Here's how the part is built. I have some questions about the finished solid (model axes, mm). Face numbers are marked on the shaded views. Round coordinates to 2 decimals unless told otherwise and drop trailing zeros. Loops run counter-clockwise (first coordinate to the right, second up) from the corner with the lowest first, then second, coordinate; pieces in that order, holes last. Notation, with made-up numbers: M -12,-16.75 L 20,-16.75 A19 ccw 20,-9.75 Z; hole C 6.5,84 d8. An arc over 180 degrees is marked long. Use a Markdown table: item, result.
```python
from build123d import *

# Parameters (mm, degrees)
SKETCH1_W           = 43.6
SKETCH1_H           = 20
BOSS_EXTRUDE1_DEPTH = 3
SKETCH4_R           = 14
CUT_EXTRUDE1_DEPTH  = 4
FILLET1_R           = 5
SKETCH3_W           = 3
SKETCH3_H           = 5
BOSS_EXTRUDE2_DEPTH = 3
LPATTERN1_COUNT     = 2
LPATTERN1_PITCH     = 30


with BuildPart() as part:
    # Sketch1 → Boss-Extrude1 (new body)
    with BuildSketch(Plane(origin=(0, 0, 0), x_dir=(0, 0, -1), z_dir=(1, 0, 0))):
        with Locations((-8.2, -1.75)):
            Rectangle(SKETCH1_W, SKETCH1_H)
    extrude(amount=BOSS_EXTRUDE1_DEPTH)

    # Sketch4 → Cut-Extrude1 (cut, through all)
    with BuildSketch(Plane(origin=(3, 0, 0), x_dir=(0, 0, -1), z_dir=(1, 0, 0))):
        with Locations((-8.2, 8.25)):
            Circle(SKETCH4_R)
    extrude(amount=-CUT_EXTRUDE1_DEPTH, mode=Mode.SUBTRACT)

    # Fillet1
    fillet1_edges = [part.edges().sort_by_distance(p)[0] for p in [
        (1.5, 8.25, 30),
        (1.5, 8.25, -13.6),
    ]]
    fillet(fillet1_edges, radius=FILLET1_R)

    # Sketch3 → Boss-Extrude2 (add)
    with BuildSketch(Plane.XZ.offset(11.75)):
        with Locations((1.5, 25)):
            Rectangle(SKETCH3_W, SKETCH3_H)
    boss_extrude2 = extrude(amount=BOSS_EXTRUDE2_DEPTH)

    # LPattern1: Boss-Extrude2 ×2
    with Locations(*[(0, 0, -i * LPATTERN1_PITCH) for i in range(1, LPATTERN1_COUNT)]):
        add(boss_extrude2)


solid = part.part
```
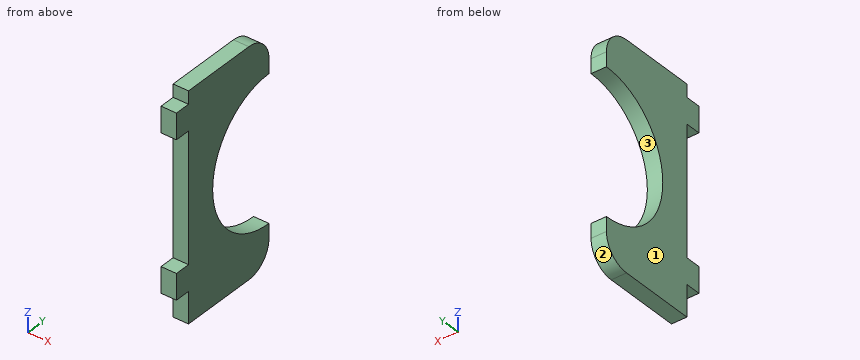
Q1. Imagine slicing it at C-C, the plane z = 8.2. Please give me the cut outline in (x, y), then the cut area to 3 significant figures.
Return value:
| item | result |
|---|---|
| outline | M 0,-11.75 L 3,-11.75 L 3,-5.75 L 0,-5.75 Z |
| area | 18.0 mm^2 |
Q2. We'd pull the mould along Z, two halves only. Please class the marked faces 1, 2 and 3: pulls with the +Z half, pulls with the -Z half, needs draft (parallel to the pull), parting line crosses it, or undercut.
Return value:
| item | result |
|---|---|
| face 1 | needs draft |
| face 2 | pulls with the -Z half |
| face 3 | undercut |
Q3. Imagine slicing it at D-D, the plane z = 16. Please give me the cut outline in (x, y).
Return value:
| item | result |
|---|---|
| outline | M 0,-11.75 L 3,-11.75 L 3,-3.38 L 0,-3.38 Z |
Q4. Will these pins go through, and if not, where does the flat tip stop? P1, Ø0.9, axis at x = 1.5, y = -13.5, coming from the +Z side; P2, Ø6, axis at y = 0.5, z = 18.5, coming from the +X side; P3, Ø1.5, axis at x = 2, z = 4, coming from the -Y side.
Return value:
| item | result |
|---|---|
| P1 | stops at z = 27.5 |
| P2 | stops at x = 3 |
| P3 | stops at y = -11.75 |
Q5. I need wall thicknesses on line 1 (Z direction, x = 0.3, y = 2.75); line 2 (Z direction, x = 1.5, y = -0.5); line 3 (Y direction, x = 0.8, z = -12). Which ranges of each line are inside material? Lowest first, please. Write a range as from..to.
Return value:
| item | result |
|---|---|
| line 1 | z = -13.6..-4.67, 21.07..30 |
| line 2 | z = -13.6..-2.73, 19.13..30 |
| line 3 | y = -11.75..6.92 |
Q6. Imagine slicing it at B-B, the plane y = -2.5. Please give me the cut outline in (x, z).
Return value:
| item | result |
|---|---|
| outline | M 0,-13.6 L 3,-13.6 L 3,-0.77 L 0,-0.77 Z; M 0,17.17 L 3,17.17 L 3,30 L 0,30 Z |
Q7. Imagine slicing it at A-A, the plane x = 0.4. Please give me the cut outline in (y, z), then the cut area to 3 significant figures.
Return value:
| item | result |
|---|---|
| outline | M -14.75,-7.5 L -11.75,-7.5 L -11.75,-13.6 L 3.25,-13.6 A5 ccw 8.25,-8.6 L 8.25,-5.8 A14 cw 8.25,22.2 L 8.25,25 A5 ccw 3.25,30 L -11.75,30 L -11.75,27.5 L -14.75,27.5 L -14.75,22.5 L -11.75,22.5 L -11.75,-2.5 L -14.75,-2.5 Z |
| area | 583 mm^2 |
